from build123d import *

# Parameters (mm, degrees)
F1_DEPTH    = 2.05
F2_R        = 1.778
F3_T1_DEPTH = 21.8600313558
F3_T3_DEPTH = 20.039287103


# Not quite as in the source:
# - a fillet or chamfer that OpenCascade refuses, or shapes differently, is made with other operations: its cross-section is extruded or revolved along the edge and cut away or added


with BuildPart() as f1:
    # F0 (on Front) → F1 (new body, symmetric)
    with BuildSketch(Plane.XZ):
        with BuildLine():
            Line((10.9602659295, 4.8513999983), (9.6458090239, 4.8513999983))
            add(Edge.make_bspline(
                [(9.6458090239, 4.8513999983), (7.4316049079, 4.8513999983), (5.2174007918, 4.8513999983), (3.0031966758, 4.8513999983)],
                knots=[0, 0, 0, 0, 1, 1, 1, 1], degree=3))
            Line((3.0031966758, 4.8513999983), (1.6934335208, 4.8513999983))
            Line((1.6934335208, 4.8513999983), (1.0692595786, 0.6714852005))
            Line((1.0692595786, 0.6714852005), (0.1693212299, 0.6714852005))
            Line((0.1693212299, 0.6714852005), (-6.1e-09, 0.2293704145))
            Line((-6.1e-09, 0.2293704145), (2.07e-08, -13.0581609413))
            add(Edge.make_bspline(
                [(2.07e-08, -13.0581609413), (0.2048945317, -13.5783853515), (0.7213722482, -13.7736584116)],
                knots=[5.4605557212, 5.4605557212, 5.4605557212, 6.2831853072, 6.2831853072, 6.2831853072], degree=2, weights=[1, 0.9165959415, 1]))
            Line((0.7213722482, -13.7736584116), (0.9610938358, -13.8642938587))
            Line((0.9610938358, -13.8642938587), (2.1238978538, -18.0086))
            Line((2.1238978538, -18.0086), (3.4693217803, -18.0086))
            add(Edge.make_bspline(
                [(9.646094231, -18.0086), (7.5871700808, -18.0086), (5.5282459306, -18.0086), (3.4693217803, -18.0086)],
                knots=[0, 0, 0, 0, 1, 1, 1, 1], degree=3))
            Line((9.646094231, -18.0086), (10.9602659326, -18.0086))
            Line((10.9602659326, -18.0086), (11.6790564953, -13.801625983))
            Line((11.6790564953, -13.801625983), (12.7507999945, -13.4755201564))
            Line((12.7507999945, -13.4755201564), (12.7507999945, 0.2137669466))
            Line((12.7507999945, 0.2137669466), (11.679056502, 0.6762536924))
            Line((11.679056502, 0.6762536924), (10.9602659295, 4.8513999983))
        make_face()
    extrude(amount=F1_DEPTH, both=True)

    # F2
    f2_edges = [f1.edges().sort_by_distance(p)[0] for p in [
        (1.381347, -2.05, 2.761443),
        (1.381347, 2.05, 2.761443),
        (11.319661, -2.05, 2.763827),
        (11.319661, 2.05, 2.763827),
        (11.319661, -2.05, -15.905113),
        (1.542496, -2.05, -15.936447),
        (11.319661, 2.05, -15.905113),
        (1.542496, 2.05, -15.936447),
    ]]
    fillet(f2_edges, radius=F2_R)

    # F3: fillet of radius 1.27 on 4 edges, made by hand

    # F3_s2 → F3_t1 (cut)
    with BuildSketch(Plane.XY.offset(-16.2331609413)):
        with BuildLine():
            ThreePointArc((1.269999983, -2.05), (0.3719743709, -1.6780256121), (-1.7e-08, -0.78))
            Line((-1.7e-08, -0.78), (-1.7e-08, -2.05))
            Line((-1.7e-08, -2.05), (1.269999983, -2.05))
        make_face()
        with BuildLine():
            ThreePointArc((1.269999983, 2.05), (0.3719743709, 1.6780256121), (-1.7e-08, 0.78))
            Line((-1.7e-08, 0.78), (-1.7e-08, 2.05))
            Line((-1.7e-08, 2.05), (1.269999983, 2.05))
        make_face()
    extrude(amount=F3_T1_DEPTH, mode=Mode.SUBTRACT)

    # F3_s4 → F3_t3 (cut)
    with BuildSketch(Plane.XY.offset(-16.6505201564)):
        with BuildLine():
            ThreePointArc((11.4807999945, 2.05), (12.3788256067, 1.6780256121), (12.7507999945, 0.78))
            Line((12.7507999945, 0.78), (12.7507999945, 2.05))
            Line((12.7507999945, 2.05), (11.4807999945, 2.05))
        make_face()
        with BuildLine():
            ThreePointArc((11.4807999945, -2.05), (12.3788256067, -1.6780256121), (12.7507999945, -0.78))
            Line((12.7507999945, -0.78), (12.7507999945, -2.05))
            Line((12.7507999945, -2.05), (11.4807999945, -2.05))
        make_face()
    extrude(amount=F3_T3_DEPTH, mode=Mode.SUBTRACT)


solid = f1.part
Check sheet for the modelled part. Datum: model origin and axes. Units: mm. A direction names the side the tool comes from. Give positions to 0.01 mm unless a question says otherwise; leave off trailing zeros. Write each loop counter-clockwise with the first axis right and the second up, starting at its lowest first coordinate (ties: lowest second). Pieces come first, ordered by that corner, then holes. Notation, with made-up numbers: (-8.5, -39) -> (-0.5, -39) arc R7 ccw to (-0.5, -29) -> close; hole circle Ø11 at (14, 69). An arc over 180 degrees is marked (long way). Write item = value, one per line.
Item 1: Tool access check on faces 1 (the flat face through (11.93, -0.03, 0.57)), 2 (the cylindrical face through (12.369, -1.688, -6.652)), 3 (the flat face through (11.904, -0.029, -13.733)). Record the directions out of +Z, -Z, +X, -X, +Y, -Y that give a thin tool (end or side, any length) a straight path to the whole face; none if there is none.
Output:
face_1 = +Z, +X
face_2 = +Z, -Z, +X, -Y
face_3 = -Z, +X
Item 2: Sectioned sample at A-A on z = -3. Record the boundary of the cut face in (x, y).
Output:
outline = (0, -0.78) arc R1.27 ccw to (1.27, -2.05) -> (11.48, -2.05) arc R1.27 ccw to (12.75, -0.78) -> (12.75, 0.78) arc R1.27 ccw to (11.48, 2.05) -> (1.27, 2.05) arc R1.27 ccw to (0, 0.78) -> close
Item 3: Scan lines: probe 1 along X at (y, z) = (-0.85, -3); probe 2 along X at (y, z) = (1.65, -3); probe 3 along Z at (x, y) = (11.75, -0.35). Record each from-to range of solid material in increasing order. Write a range as from..to.
Output:
probe_1 = 0..12.75
probe_2 = 0.34..12.41
probe_3 = -13.78..0.65
